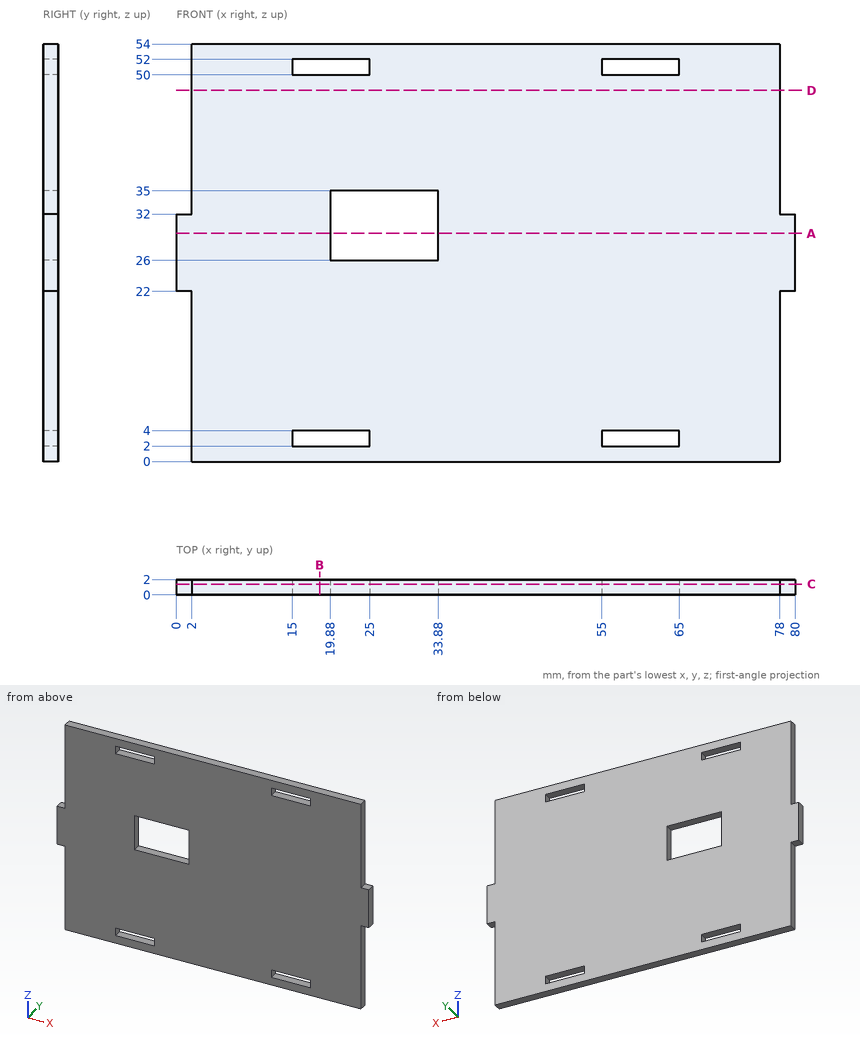
Design review of the part shown in the three views and the two pictorial views. Dimensions are in mm from the part's minimum x, y and z. Round coordinates to 2 decimals unless told otherwise and drop trailing zeros. Write each loop counter-clockwise with the first axis right and the second up, starting at its lowest first coordinate (ties: lowest second). Pieces come first, ordered by that corner, then holes. Notation, with made-up numbers: (2.25, 18) - (25.25, 18) arc R19 cw to (25.25, 42) - close; hole circle Ø3 at (-6.75, 50). An arc over 180 degrees is marked (long way). Return JSON: item names as keys, results as strings. Group by question number.
Item 1: We need section C-C on y = 1.4. Give the number of separate pieces and of enclosed holes in the cut face, and give its area (3 significant figures).
Item 2: For probe 1 along Z at (x, y) = (63, 0.75); probe 2 along Z at (x, y) = (22.5, 1.35); probe 3 along X at (y, z) = (1.75, 10.5), list the stretches that pass through material, from the lowest coordinate up. Write a range as [from, to].
Item 3: We need section B-B on x = 18.5. Write out the cut boundary in (y, z), and give its area (3 significant figures).
Item 4: Insertion check: P1, Ø1, axis at y = 1.5, z = 2.5, coming from the -X side; P2, Ø0.6, axis at x = 1.5, y = 1.5, coming from the -Z side; P3, Ø0.6, axis at y = 0.5, z = 42.5, coming from the +X side. Each pin has a flat end and moves straight along its axis. Give the tip position at first contact, or say it passes through.
Item 5: We need section A-A on z = 29.5. Write out the cut boundary in (x, y).
Item 6: We need section D-D on z = 48. Write out the cut boundary in (x, y), and give its area (3 significant figures).
Model answer:
{
 "1": {"separate pieces": "1", "enclosed holes": "5", "area": "3,940 mm²"},
 "2": {"probe 1": "z = [0, 2], [4, 50], [52, 54]", "probe 2": "z = [0, 2], [4, 26], [35, 50], [52, 54]", "probe 3": "x = [2, 78]"},
 "3": {"outline": "(0, 0) - (2, 0) - (2, 2) - (0, 2) - close; (0, 4) - (2, 4) - (2, 50) - (0, 50) - close; (0, 52) - (2, 52) - (2, 54) - (0, 54) - close", "area": "100 mm²"},
 "4": {"P1": "stops at x = 2", "P2": "stops at z = 22", "P3": "stops at x = 78"},
 "5": {"outline": "(0, 0) - (19.88, 0) - (19.88, 2) - (0, 2) - close; (33.88, 0) - (80, 0) - (80, 2) - (33.88, 2) - close"},
 "6": {"outline": "(2, 0) - (78, 0) - (78, 2) - (2, 2) - close", "area": "152 mm²"}
}
